Here's how the part is built. I have some questions about the finished solid (model axes, mm). Round coordinates to 2 decimals unless told otherwise and drop trailing zeros. Write each loop counter-clockwise with the first axis right and the second up, starting at its lowest first coordinate (ties: lowest second). Pieces come first, ordered by that corner, then holes. Notation, with made-up numbers: (38, -29.75) -> (90, -29.75) arc R30 cw to (90, -7.75) -> close; hole circle Ø5 at (-9, 38). An arc over 180 degrees is marked (long way). Answer as CSV lines item,"result".
Autodesk Inventor part; units mm, degrees
ref_plane "YZ Plane" through (0, 0, 0) normal (1, 0, 0) x (0, 1, 0)
ref_plane "XZ Plane" through (0, 0, 0) normal (0, 1, 0) x (-1, 0, 0)
ref_plane "XY Plane" through (0, 0, 0) normal (0, 0, 1) x (1, 0, 0)
sketch "Sketch1" plane through (0, 0, 0) normal (0, 1, 0) x (-1, 0, 0)
  line L0 (3.9616, 0) -> (-12.9611, 0)
  line L1 (-12.9611, 0) -> (-12.9611, -3)
  line L2 (-12.9611, -3) -> (-0.9611, -3)
  line L3 (-12.9611, -3) -> (-0.9611, -3) construction
  line L4 (-0.9611, -3) -> (-0.9611, -11.5)
  line L5 (-0.9611, -11.5) -> (3.0389, -11.5)
  arc A0 (3.0389, -11.5) -> (3.9616, 0) centre (-48.7312, -1.5591) ccw
  line L6 (61.7439, 0) -> (-67.1437, 0)
  arc A1 (3.3616, 0) -> (3.8723, -5) centre (43.3314, 1.556) ccw
  line L7 (3.8723, -5) -> (7.1647, 0)
  line L8 (7.1647, 0) -> (3.3616, 0)
  point P0 (0, 0)
  dimension "d1" = 3
  dimension "d2" = 90
  dimension "d3" = 12
  dimension "d5" = 8.5
  dimension "d6" = 4
  dimension "d11" = 0
  dimension "d14" = 0.6
  dimension "d16" = 5
  dimension "d17" = 40
revolve "Revolution1" add sketch "Sketch1" angle 360 about axis through (-10, 0, 0) along (1, 0, 0) contours A0 A1 L0 | A1 A0 L5 L4 L2 L1 L0
fillet "Fillet1" radius 2.3 2 edges at (-3.0389, 0, 11.5) (0.9611, 0, 11.5)
sketch "Sketch2" plane through (12.9611, 0, 0) normal (1, 0, 0) x (0, 0, -1)
  circle A0 centre (0, 0) radius 3
  line L0 (1.9, 1.9) -> (-1.9, 1.9)
  line L1 (-1.9, 1.9) -> (-1.9, -1.9)
  line L2 (-1.9, -1.9) -> (1.9, -1.9)
  line L3 (1.9, -1.9) -> (1.9, 1.9)
  line L4 (1.9, 1.9) -> (-1.9, -1.9) construction
  line L5 (-1.9, 1.9) -> (1.9, -1.9) construction
  dimension "d9" = 3.8
  dimension "d10" = 3.8
extrude "Extrusion1" cut sketch "Sketch2" against normal blind 3 contours L3 L2 L1 L0
revolve "Revolution2" cut sketch "Sketch1" angle 360 about axis through (-10, 0, 0) along (1, 0, 0) contours A0 A1 L0 | L6 L7 A0
properties part number "joystick_nibble"
Item 1: Will these pins go through, and if not, where does the flat tip stop? pin 1 (3.5 mm diameter, centred on x = 11, y = -1, fed in from +Z); pin 2 (1.5 mm diameter, centred on y = 6.5, z = 4, fed in from -X); pin 3 (1.5 mm diameter, centred on x = 11, z = 0, fed in from +Y).
Results found:
pin 1,"stops at z = 3"
pin 2,"stops at x = -3.72"
pin 3,"stops at y = 3"
Item 2: Suppose I cut it at A-A, the plane x = 3.5. List the corners of the cut face in (y, z) for me.
Results found:
outline,"circle Ø6 at (0, 0)"
Item 3: If we mould it in two halves opening along Z, with no side actions, what happens to faces 1 (the cylindrical face through (7, 0, 3)), 2 (the flat face through (9.961, 0, 0)), 3 (the flat face through (0.961, 0.1, 3.2))? For each: pulls with the +Z half, pulls with the -Z half, needs draft (parallel to the pull), parting line crosses it, or undercut.
Results found:
face 1,"parting line crosses it"
face 2,"undercut"
face 3,"needs draft"
Item 4: I need wall thicknesses on L1, parallel to X at y = 0.5, z = -5; L2, parallel to Y at x = 7.75, z = 0.75; L3, parallel to Y at x = 5.5, z = -0.5. Which ranges of each line are inside material? Lowest first, please.
Results found:
L1,"x = -3.87 to 0.96"
L2,"y = -2.9 to 2.9"
L3,"y = -2.96 to 2.96"
